```python
from build123d import *

# Parameters (mm, degrees)
EXTRUDE002_DEPTH           = 3
EXTRUDE002_PLACEMENT_ANGLE = 120
EXTRUDE001_DEPTH           = 3
CHAMFER_SIZE               = 1
CYLINDER001_R              = 4.05
CYLINDER001_DEPTH          = 10
CYLINDER002_W              = 9.5
CYLINDER002_H              = 8
CYLINDER002_ANGLE          = 54
CYLINDER_W                 = 9.5
CYLINDER_H                 = 1
CYLINDER_ANGLE             = 120


with BuildPart() as extrude002:
    # Sketch001 (on Face11 of Cut002) → Extrude002 (new body)
    with BuildSketch(Plane.XY.offset(8)):
        Polygon((13.2649878575, 2.1), (9.2649878575, 2.1), (7.7, 0), (9.2649878575, -2.1), (13.2649878575, -2.1), align=None)
    extrude(amount=-EXTRUDE002_DEPTH)


with BuildPart() as extrude002_1:
    # Extrude002 placement: moved
    add(extrude002.part.moved(Location((0, 0, -7))).rotate(Axis((0, 0, -7), (0, 0, 1)), EXTRUDE002_PLACEMENT_ANGLE))


with BuildPart() as chamfer_body:
    # Sketch001 (on Face11 of Cut002) → Extrude001 (new body)
    with BuildSketch(Plane.XY.offset(8)):
        Polygon((13.2649878575, 2.1), (9.2649878575, 2.1), (7.7, 0), (9.2649878575, -2.1), (13.2649878575, -2.1), align=None)
    extrude(amount=-EXTRUDE001_DEPTH)

    # Chamfer
    chamfer_edges = [chamfer_body.edges().sort_by_distance(p)[0] for p in [
        (13.264988, 2.1, 6.5),
        (13.264988, -2.1, 6.5),
    ]]
    chamfer(chamfer_edges, length=CHAMFER_SIZE)


with BuildPart() as cylinder001:
    # Cylinder001 → Cylinder001 (new body)
    with BuildSketch(Plane.XY):
        Circle(CYLINDER001_R)
    extrude(amount=CYLINDER001_DEPTH)


with BuildPart() as cylinder002:
    # Cylinder002 → Cylinder002 (revolve)
    with BuildSketch(Plane.XZ):
        with Locations((4.75, 4)):
            Rectangle(CYLINDER002_W, CYLINDER002_H)
    revolve(axis=Axis((0, 0, 0), (0, 0, 1)), revolution_arc=CYLINDER002_ANGLE)


with BuildPart() as cut003:
    # Cylinder → Cylinder (revolve)
    with BuildSketch(Plane.XZ):
        with Locations((4.75, 0.5)):
            Rectangle(CYLINDER_W, CYLINDER_H)
    revolve(axis=Axis((0, 0, 0), (0, 0, 1)), revolution_arc=CYLINDER_ANGLE)

    # Fusion: union Cylinder002
    add(cylinder002.part)

    # Cut002: cut Cylinder001
    add(cylinder001.part, mode=Mode.SUBTRACT)

    # Fusion001: union Chamfer body
    add(chamfer_body.part)

    # Cut003: cut Extrude002
    add(extrude002_1.part, mode=Mode.SUBTRACT)


solid = cut003.part
```
CAD build for the part. Positions are in the model's coordinates, mm. A direction names the side the tool comes from. Give positions to 0.01 mm unless a question says otherwise; leave off trailing zeros. Order: outer loops, then holes, each group sorted by start corner. A loop starts at its lowest first (then second) coordinate and runs counter-clockwise, first axis right, second up. Notation, with made-up numbers: M 81,46.25 L 110,46.25 A13 cw 110,58.25 Z; hole C 60,66 d10. An arc over 180 degrees is marked long. Put each result on its own line as item: value. Start each with the question number.
(1) Drill centre lines: line 1 along Z through (x, y) = (2.25, 6); line 2 along Y through (x, z) = (11.75, 7); line 3 along Y through (x, z) = (5.5, 1.5). Where is each one in solid material? Low to high.
(2) Saw through at A-A, the plane z = 6.75. Write the cut outline in (x, y), then the cut area to 3 significant figures.
(3) Which spindle directions (+Z, -Z, +X, -X, +Y, -Y) get a long thin tool onto all of the face, cutting with end or side? Do faces 1 (the flat face through (3.96, 5.45, 4.55)), 2 (the flat face through (11, 2.1, 7)), 3 (the flat face through (7, 0, 4)). Say none if no direction does.
(4) Flat gauge pins, fed straight in: pin 1 Ø5 at (x, y) = (1.5, 6.5) entering from +Z; pin 2 Ø2 at (x, z) = (5.5, 4) entering from -Y; pin 3 Ø0.9 at (x, z) = (11.5, 6.5) entering from +Y. Where does each tip first touch, or does it go through?
(5) Saw through at C-C, the plane x = 11.75. Write the cut outline in (y, z).
(6) Saw through at D-D, the plane z = 0.5. Write the cut outline in (x, y) (3 decimals).
(7) Saw through at B-B, the plane y = 6. Write the cut outline in (x, z), then the cut area to 3 significant figures.
Check result:
1. line 1: z = 0 to 1
1. line 2: y = -2.1 to 2.1
1. line 3: y = 0 to 7.57
2. outline: M 2.38,3.28 A4.05 cw 4.05,0 L 7.7,0 L 9.26,-2.1 L 12.26,-2.1 L 13.26,-1.1 L 13.26,1.1 L 12.26,2.1 L 9.26,2.1 A9.5 ccw 5.58,7.69 Z
2. area: 51.9 mm2
3. face 1: +Z, -X, +Y
3. face 2: +Z, -Z, +X, +Y
3. face 3: -Z, -X, -Y
4. pin 1: stops at z = 1
4. pin 2: stops at y = 0
4. pin 3: stops at y = 2.1
5. outline: M -2.1,5 L 2.1,5 L 2.1,8 L -2.1,8 Z
6. outline: M -3.85,6.668 L -2.025,3.507 A4.05 cw 4.05,0 L 9.5,0 A9.5 ccw -2.814,9.074 Z
7. outline: M -3.46,0 L 7.37,0 L 7.37,8 L 4.36,8 L 4.36,1 L -3.46,1 Z
7. area: 31.9 mm2
